Design review of the part built by this model. Coordinates are the model's own, in mm. Face numbers are marked on the shaded views. Round coordinates to 2 decimals unless told otherwise and drop trailing zeros. Order: outer loops, then holes, each group sorted by start corner. A loop starts at its lowest first (then second) coordinate and runs counter-clockwise, first axis right, second up. Notation, with made-up numbers: M 26,-34 L 41,-34 A25 ccw 41,-9 Z; hole C 82,26.5 d3. An arc over 180 degrees is marked long. Write item = value, one per line. Start each with the question number.
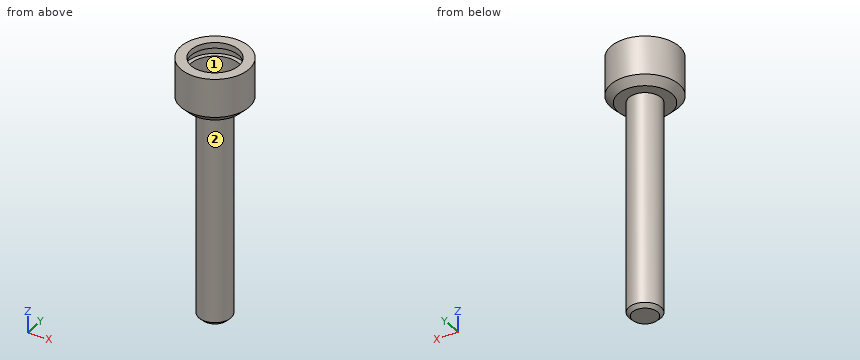
```python
from build123d import *

# Parameters (mm, degrees)
F0_R     = 9.525
F1_DEPTH = 12.7
F2_R     = 6.6675
F3_DEPTH = 9.525
F4_W     = 1.1938
F4_H     = 2.2352
F7_SIZE  = 2
F8_R     = 4.485
F9_DEPTH = 60
F10_SIZE = 1


# Not quite as in the source:
# - the program builds the solid bodies; features that only make, move or delete a surface that nothing else refers to are left out


with BuildPart() as f1:
    # F0 (on Top) → F1 (new body)
    with BuildSketch(Plane.XY):
        Circle(F0_R)
    extrude(amount=F1_DEPTH)

    # F2 (on face) → F3 (cut)
    with BuildSketch(Plane.XY.offset(12.7)):
        Circle(F2_R)
    extrude(amount=-F3_DEPTH, mode=Mode.SUBTRACT)

    # F4 (on Front) → F5 (revolve, cut)
    with BuildSketch(Plane.XZ):
        with Locations((7.2644, 9.9949)):
            Rectangle(F4_W, F4_H)
    revolve(axis=Axis((0, 0, 19.0221574157), (0, 0, 1)), mode=Mode.SUBTRACT)

    # F7
    f7_edges = [f1.edges().sort_by_distance(p)[0] for p in [
        (-9.525, 0, 0),
    ]]
    chamfer(f7_edges, length=F7_SIZE)

    # F8 (on face) → F9 (join)
    with BuildSketch(Plane(origin=(0, 0, 0), x_dir=(1, 0, 0), z_dir=(0, 0, -1))):
        Circle(F8_R)
    extrude(amount=F9_DEPTH)

    # F10
    f10_edges = [f1.edges().sort_by_distance(p)[0] for p in [
        (-4.485, 0, -60),
    ]]
    chamfer(f10_edges, length=F10_SIZE)


solid = f1.part
```
(1) Insertion check: pin 1 (8 mm diameter, centred on x = 0, y = 0, fed in from +Z) (3 decimals); pin 2 (3 mm diameter, centred on x = -0.5, z = -51, fed in from +Y) (3 decimals); pin 3 (4 mm diameter, centred on y = -0.5, z = -17.5, fed in from +X) (3 decimals). Each pin has a flat end and moves straight along its axis. Give the tip position at first contact, or say it passes through.
(2) For line 1 along Y through (x, z) = (0, 12.3) (1 decimal); line 2 along Y through (x, z) = (0, 9.6) (3 decimals); line 3 along Z through (x, y) = (4.75, -5.5), list the stretches that pass through material, from the lowest coordinate up. Write a range as [from, to].
(3) Consider section C-C, the plane z = -53. Write out the cut boundary in (x, y) (3 decimals).
(4) Consider section A-A, the plane y = 0. Write out the cut boundary in (x, z) (1 decimal).
(5) Draft analysis for pull direction X (two halves, no side actions). For the marked faces 1 and 2, state which applies: pulls with the +X half, pulls with the -X half, needs draft (parallel to the pull), parting line crosses it, or undercut.
Completed:
q1.pin_1 = 3.175
q1.pin_2 = 4.485
q1.pin_3 = 4.485
q2.line_1 = [-9.5, -6.7], [6.7, 9.5]
q2.line_2 = [-9.525, -7.861], [7.861, 9.525]
q2.line_3 = [0, 8.88], [11.11, 12.7]
q3.outline = C 0,0 d8.97
q4.outline = M -9.5,2 L -7.5,0 L -4.5,0 L -4.5,-59 L -3.5,-60 L 3.5,-60 L 4.5,-59 L 4.5,0 L 7.5,0 L 9.5,2 L 9.5,12.7 L 6.7,12.7 L 6.7,11.1 L 7.9,11.1 L 7.9,8.9 L 6.7,8.9 L 6.7,3.2 L -6.7,3.2 L -6.7,8.9 L -7.9,8.9 L -7.9,11.1 L -6.7,11.1 L -6.7,12.7 L -9.5,12.7 Z
q5.face_1 = undercut
q5.face_2 = parting line crosses it
